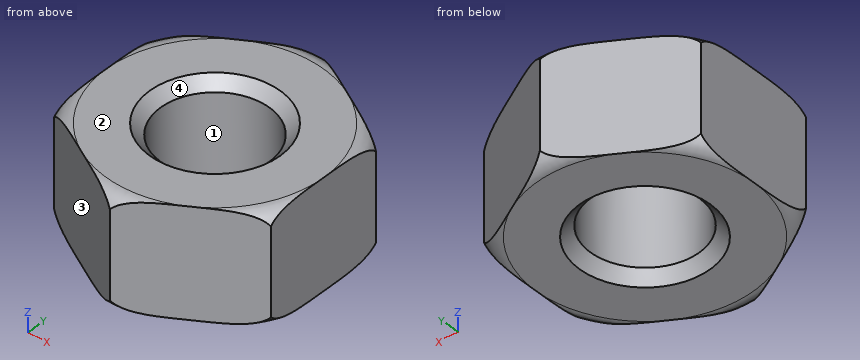
```python
from build123d import *

# Parameters (mm, degrees)
F2_R     = 6.562274
F3_DEPTH = 12.5


with BuildPart() as f1:
    # F0 (on Front) → F1 (revolve)
    with BuildSketch(Plane.XZ):
        with BuildLine():
            Line((-2.5, -2), (-2.5, 0))
            Line((-2.5, 0), (-2.5, 2))
            Line((-2.5, 2), (-3, 2.5))
            Line((-3, 2.5), (-5, 2.5))
            ThreePointArc((-5, 2.5), (-5.460518, 2.364117), (-5.773503, 2))
            Line((-5.773503, 2), (-5.773503, 0))
            Line((-5.773503, 0), (-5.773503, -2))
            ThreePointArc((-5.773503, -2), (-5.460518, -2.364117), (-5, -2.5))
            Line((-5, -2.5), (-3, -2.5))
            Line((-3, -2.5), (-2.5, -2))
        make_face()
    revolve(axis=Axis((0, 0, 4.430122), (0, 0, 1)))

    # F2 (on Top) → F3 (cut, symmetric)
    with BuildSketch(Plane.XY):
        Circle(F2_R)
        Polygon((0, 5.773503), (5, 2.886751), (5, -2.886751), (0, -5.773503), (-5, -2.886751), (-5, 2.886751), align=None, mode=Mode.SUBTRACT)
    extrude(amount=F3_DEPTH, both=True, mode=Mode.SUBTRACT)


solid = f1.part
```
Can you work these out from the model? Positions are in its coordinate system, mm. Face numbers are marked on the shaded views. Give positions to 0.01 mm unless a question says otherwise; leave off trailing zeros. Loops run counter-clockwise (first coordinate to the right, second up) from the corner with the lowest first, then second, coordinate; pieces in that order, holes last. Notation, with made-up numbers: M 79.5,-19 L 121.5,-19 A24 cw 121.5,-3 Z; hole C 23.5,18 d2. An arc over 180 degrees is marked long. Answer in a Markdown table with one row per item.
1. Thinking about a two-plate mould opening in X: for the marked faces 1, 2, 3 and 4, which applies, released by +X, released by -X, zero draft, split by the parting line, or undercut?
Taken from the geometry:
| item | result |
|---|---|
| face 1 | undercut |
| face 2 | zero draft |
| face 3 | released by -X |
| face 4 | undercut |
2. For pin 1 Ø2 at (x, z) = (3, 0) entering from +Y; pin 2 Ø3 at (x, z) = (2, -1) entering from -Y; pin 3 Ø1.5 at (x, z) = (-0.5, -1) entering from -Y; pin 4 Ø5 at (x, y) = (-1, -2.5) entering from +Z, each with a flat end and sliding along its axis, tell me the tip position at first contact or that it passes through.
Taken from the geometry:
| item | result |
|---|---|
| pin 1 | stops at y = 4.62 |
| pin 2 | stops at y = -5.48 |
| pin 3 | stops at y = -5.77 |
| pin 4 | stops at z = 2.5 |
3. If I drill on line 1 along X through (y, z) = (0, 0.9); line 2 along Y through (x, z) = (2, 0.05); line 3 along Y through (x, z) = (0.5, -1.1), over which ranges is the centre line in solid material (lowest first)?
Taken from the geometry:
| item | result |
|---|---|
| line 1 | x = -5 to -2.5, 2.5 to 5 |
| line 2 | y = -4.62 to -1.5, 1.5 to 4.62 |
| line 3 | y = -5.48 to -2.45, 2.45 to 5.48 |
4. Suppose I cut it at A-A on z = 0.1. Write out the boundary of the cut face in (x, y).
Taken from the geometry:
| item | result |
|---|---|
| outline | M -5,-2.89 L 0,-5.77 L 5,-2.89 L 5,2.89 L 0,5.77 L -5,2.89 Z; hole C 0,0 d5 |
